Verification items for this drawing (mm, ordinates from the low corner). A direction names the side the tool comes from. Round coordinates to 2 decimals unless told otherwise and drop trailing zeros. Loops run counter-clockwise (first coordinate to the right, second up) from the corner with the lowest first, then second, coordinate; pieces in that order, holes last. Notation, with made-up numbers: (61.25, 9.25) -> (112.25, 9.25) arc R19 ccw to (112.25, 30.25) -> close; hole circle Ø4 at (13, 43). An arc over 180 degrees is marked (long way). One line per question, with ' | ' between items.
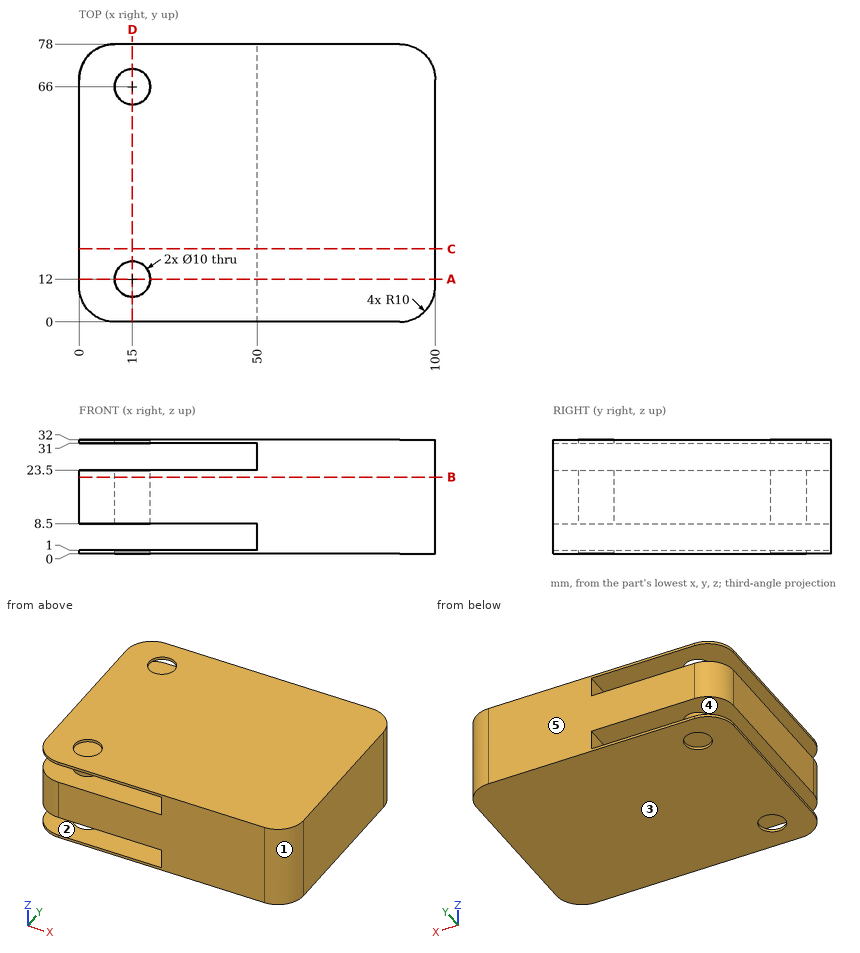
(1) Go/stop test with a flat-tipped pin: pin 1 (2 mm diameter, centred on y = 30.5, z = 5, fed in from -X). Record where the tip stops, or that it passes through.
Answer:
pin 1: stops at x = 50
(2) Set-up check for the marked faces 4 and 5: record each of +Z, -Z, +X, -X, +Y, -Y from which the full face is reachable in a straight line by a thin tool's end or side.
Answer:
face 4: -X, +Y, -Y | face 5: +Z, -Z, +X, -X, +Y
(3) Scan lines: probe 1 along Z at (x, y) = (37, 48); probe 2 along Y at (x, z) = (15, 0.3); probe 3 along X at (y, z) = (66, 17.75). Record each from-to range of solid material in increasing order.
Answer:
probe 1: z = 0 to 1, 8.5 to 23.5, 31 to 32 | probe 2: y = 0 to 7, 17 to 61, 71 to 78 | probe 3: x = 0 to 10, 20 to 100
(4) Sectioned sample at A-A, the plane y = 12. Record the cut outline in (x, z).
Answer:
outline: (0, 0) -> (10, 0) -> (10, 1) -> (0, 1) -> close; (0, 8.5) -> (10, 8.5) -> (10, 23.5) -> (0, 23.5) -> close; (0, 31) -> (10, 31) -> (10, 32) -> (0, 32) -> close; (20, 0) -> (100, 0) -> (100, 32) -> (20, 32) -> (20, 31) -> (50, 31) -> (50, 23.5) -> (20, 23.5) -> (20, 8.5) -> (50, 8.5) -> (50, 1) -> (20, 1) -> close
(5) Sectioned sample at B-B, the plane z = 21.5. Record the cut outline in (x, y), and give its area (3 significant figures).
Answer:
outline: (0, 10) arc R10 ccw to (10, 0) -> (90, 0) arc R10 ccw to (100, 10) -> (100, 68) arc R10 ccw to (90, 78) -> (10, 78) arc R10 ccw to (0, 68) -> close; hole circle Ø10 at (15, 12); hole circle Ø10 at (15, 66) | area: 7,560 mm2
(6) Sectioned sample at D-D, the plane x = 15. Count the separate pieces of the cut face and the enclosed holes in it, and give its area (3 significant figures).
Answer:
separate pieces: 9 | enclosed holes: 0 | area: 986 mm2
(7) Sectioned sample at C-C, the plane y = 20.5. Record the cut outline in (x, z).
Answer:
outline: (0, 0) -> (100, 0) -> (100, 32) -> (0, 32) -> (0, 31) -> (50, 31) -> (50, 23.5) -> (0, 23.5) -> (0, 8.5) -> (50, 8.5) -> (50, 1) -> (0, 1) -> close
(8) Mould release check, pull along Z, two halves, no side actions. Record for the marked faces 1, 2 and 3: +Z half, -Z half, draft (parallel to the pull), parting line (faces both ways), or undercut.
Answer:
face 1: draft | face 2: undercut | face 3: -Z half
